Geometry check sheet. Reference: the model listing, model coordinates, mm. A direction names the side the tool comes from. Coordinates: 2 decimals unless noted, no trailing zeros. Order: outer loops, then holes, each group sorted by start corner. A loop starts at its lowest first (then second) coordinate and runs counter-clockwise, first axis right, second up. Notation, with made-up numbers: M -13,49.25 L 3,49.25 A29 ccw 3,73.25 Z; hole C 57.25,28 d8. An arc over 180 degrees is marked long. One line per item, written item: value. Start each with the question number.
1) Access from +Z, -Z, +X, -X, +Y, -Y to the whole of each face (thin tool, end or side, straight path). Record for faces 1 (the flat face through (0, -108, 30)), 2 (the flat face through (0, -354, -40)), 3 (the flat face through (0, -128, -10)).
2) Go/stop test with flat-tipped pins: P1, Ø10, axis at y = -371.5, z = -0.5, coming from the +X side; P2, Ø8, axis at x = -12, y = -55, coming from the +Z side; P3, Ø24, axis at x = 4.5, z = -26, coming from the +Y side; P4, Ø10, axis at x = 12, y = -213, coming from the -Z side. Record where each tip stops, or that it passes through.
3) Thickness scan on L1, parallel to Z at x = -11, y = -61; L2, parallel to Y at x = 8.5, z = -15; L3, parallel to X at y = -392.5, z = 8.5. Record the ranges inside material, lowest first. Write a range as from..to.
4) Sectioned sample at A-A, the plane x = -2.5. Enter the section's corners in (y, z), then the cut area to 4 significant figures.
5) Sectioned sample at D-D, the plane y = -61. Enter the section's corners in (x, z), then the cut area to 3 significant figures.
6) Sectioned sample at C-C, the plane z = -16. Enter the section's corners in (x, y).
7) Sectioned sample at B-B, the plane y = -340. Enter the section's corners in (x, z), then the cut area to 3 significant figures.
```python
from build123d import *

# Parameters (mm, degrees)
F1_DEPTH = 450
F3_DEPTH = 220
F5_DEPTH = 260


with BuildPart() as f1:
    # F0 (on Front) → F1 (new body)
    with BuildSketch(Plane.XZ):
        Polygon((10, 45), (-10, 45), (-20, 0), (-15, -40), (15, -40), (20, 0), align=None)
    extrude(amount=F1_DEPTH)

    # F2 (on face) → F3 (cut)
    with BuildSketch(Plane(origin=(0, 0, 0), x_dir=(-1, 0, 0), z_dir=(0, 1, 0))):
        Polygon((-10, 45), (-13.3333333333, 30), (13.3333333333, 30), (10, 45), align=None)
    extrude(amount=-F3_DEPTH, mode=Mode.SUBTRACT)

    # F4 (on face) → F5 (cut)
    with BuildSketch(Plane(origin=(0, 0, 0), x_dir=(-1, 0, 0), z_dir=(0, 1, 0))):
        Polygon((18.75, -10), (-18.75, -10), (-15, -40), (15, -40), align=None)
    extrude(amount=-F5_DEPTH, mode=Mode.SUBTRACT)


solid = f1.part
```
Final values:
1. face 1: +Z, +X, -X, +Y
1. face 2: -Z, +X, -X, +Y, -Y
1. face 3: -Z, +X, -X, +Y
2. P1: stops at x = 20
2. P2: stops at z = 30
2. P3: stops at y = -260
2. P4: stops at z = -10
3. L1: z = -10..30
3. L2: y = -450..-260
3. L3: x = -18.11..18.11
4. outline: M -450,-40 L -260,-40 L -260,-10 L 0,-10 L 0,30 L -220,30 L -220,45 L -450,45 Z
4. area: 27,150 mm^2
5. outline: M -20,0 L -18.75,-10 L 18.75,-10 L 20,0 L 13.33,30 L -13.33,30 Z
5. area: 1,390 mm^2
6. outline: M -18,-450 L 18,-450 L 18,-260 L -18,-260 Z
7. outline: M -20,0 L -15,-40 L 15,-40 L 20,0 L 10,45 L -10,45 Z
7. area: 2,750 mm^2
